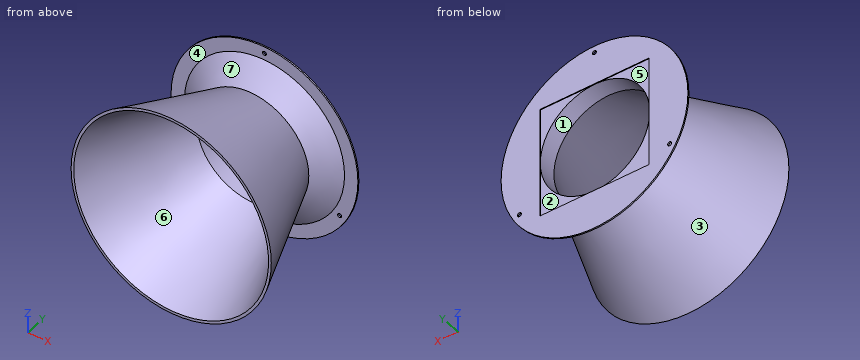
```python
from build123d import *

# Parameters (mm, degrees)
CROQUIS6_R            = 1.5
CORTAR_EXTRUIR9_DEPTH = 10
CROQUIS2_W            = 82
CROQUIS2_H            = 82
CORTAR_EXTRUIR1_DEPTH = 11.5
CROQUIS4_W            = 14
CROQUIS4_H            = 8.5
CORTAR_EXTRUIR2_DEPTH = 10.5


with BuildPart() as part:
    # Croquis1 → Revolución1 (revolve)
    with BuildSketch(Plane.XY):
        Polygon((-67.901642817, 46.97611702), (-67.901642817, 60.97611702), (-96.901642817, 60.97611702), (-96.901642817, 59.97611702), (-86.901642817, 59.97611702), (-69.901642817, 46.97611702), (-101.901642817, -33.02388298), (-99.901642817, -33.02388298), align=None)
    revolve(axis=Axis((-26.901642817, 46.97611702, 0), (0, -1, 0)))

    # Croquis6 → Cortar-Extruir9 (cut)
    with BuildSketch(Plane.XZ.offset(-59.97611702)):
        with Locations((-26.901642817, 65)):
            Circle(CROQUIS6_R)
        with Locations((29.390008429, -32.5)):
            Circle(CROQUIS6_R)
        with Locations((-83.193294063, -32.5)):
            Circle(CROQUIS6_R)
    extrude(amount=-CORTAR_EXTRUIR9_DEPTH, mode=Mode.SUBTRACT)

    # Croquis2 → Cortar-Extruir1 (cut)
    with BuildSketch(Plane(origin=(0, 71.97611702, 0), x_dir=(1, 0, 0), z_dir=(0, 1, 0))):
        with Locations((-26.901642817, 0)):
            Rectangle(CROQUIS2_W, CROQUIS2_H)
    extrude(amount=-CORTAR_EXTRUIR1_DEPTH, mode=Mode.SUBTRACT)

    # Croquis4 → Cortar-Extruir2 (cut)
    with BuildSketch(Plane.ZY.offset(-25.098357183)):
        with Locations((0, 77.22611702)):
            Rectangle(CROQUIS4_W, CROQUIS4_H)
    extrude(amount=-CORTAR_EXTRUIR2_DEPTH, mode=Mode.SUBTRACT)


solid = part.part
```
Can you work these out from the model? Positions are in its coordinate system, mm. Face numbers are marked on the shaded views. A direction names the side the tool comes from. Round coordinates to 2 decimals unless told otherwise and drop trailing zeros. Loops run counter-clockwise (first coordinate to the right, second up) from the corner with the lowest first, then second, coordinate; pieces in that order, holes last. Notation, with made-up numbers: M -16,30 L 21,30 A20 ccw 21,42 Z; hole C 88.5,27 d2. An arc over 180 degrees is marked long. Write item = value, one per line. Start each with the question number.
(1) I'm going to push flat-ended pins straight in: P1, Ø4, axis at x = -83.19, z = -32.5, coming from the -Y side; P2, Ø3, axis at y = -0.5, z = 21, coming from the -X side; P3, Ø0.5, axis at y = 60.5, z = -6.5, coming from the -X side. Where does each tip first touch, or does it pass through?
(2) Suppose I cut it at A-A on y = 42. Write out the boundary of the cut face in (x, z), plus the area to 3 significant figures.
(3) Which directions (+Z, -Z, +X, -X, +Y, -Y) give clear straight access to the entire face, cutting with the end or side of a thin tool? Please do the marked faces 5, 6 and 7.
(4) I need wall thicknesses on line 1 along Y through (x, z) = (0.5, 33.5); line 2 along Z through (x, y) = (-32, 3); line 3 along Z through (x, y) = (12, 32). Which ranges of each line are inside material? Lowest first, please.
(5) If we mould it in two halves opening along X, with no side actions, what happens to the marked faces 1, 2, 3 and 4? For each: released by +X, released by -X, zero draft, split by the parting line, or undercut.
Answer block:
q1.P1 = -18.02
q1.P2 = -86.05
q1.P3 = -96.62
q2.outline = C -26.9,0 d89.98; hole C -26.9,0 d85.98
q2.area = 553 mm²
q3.face_5 = +Y
q3.face_6 = -Y
q3.face_7 = none
q4.line_1 = 41.28 to 46.28, 47.19 to 60.48
q4.line_2 = -60.38 to -58.37, 58.37 to 60.38
q4.line_3 = -29.78 to -26.36, 26.36 to 29.78
q5.face_1 = undercut
q5.face_2 = undercut
q5.face_3 = split by the parting line
q5.face_4 = zero draft
